Geometry check sheet. Reference: the model listing, model coordinates, mm. Face numbers are marked on the shaded views. A direction names the side the tool comes from. Give positions to 0.01 mm unless a question says otherwise; leave off trailing zeros. Loops run counter-clockwise (first coordinate to the right, second up) from the corner with the lowest first, then second, coordinate; pieces in that order, holes last. Notation, with made-up numbers: (-8, 21.25) - (18, 21.25) arc R19 cw to (18, 51.25) - close; hole circle Ø9 at (38, 4.5). An arc over 180 degrees is marked (long way). Use a Markdown table: item, result. Add a question column.
1. Depth check by flat-ended pin: P1, Ø17.5, axis at x = -1.5, y = 158.5, coming from the -Z side. Enter the tip coordinate at first touch or a pass-through.
2. Cross-section at B-B on x = -0.5. Enter the section's corners in (y, z), and give its area (3 significant figures).
3. Material ranges on L1, parallel to X at y = 82, z = -1.75; L2, parallel to Z at x = 1, y = 62; L3, parallel to X at y = 168.5, z = -6.5, recorded low to high.
4. Set-up check for the marked faces 1 and 2: record each of +Z, -Z, +X, -X, +Y, -Y from which the full face is reachable in a straight line by a thin tool's end or side.
5. Cross-section at A-A on y = 31.5. Enter the section's corners in (x, z).
from build123d import *

# Parameters (mm, degrees)
RUNDUNG_DEPTH        = 250
SKIZZE2_W            = 22
SKIZZE2_H            = 3.270726357
AUSSPARUNGLAUF_DEPTH = 252.122480077


with BuildPart() as part:
    # Skizze1 → Rundung (new body)
    with BuildSketch(Plane(origin=(0, 0, 0), x_dir=(1, 0, 0), z_dir=(0, 1, 0))):
        with BuildLine():
            Line((-19.158288024, 7.5), (-22.5, 7.5))
            Line((-22.5, 7.5), (-22.5, -7.5))
            Line((-22.5, -7.5), (22.5, -7.5))
            Line((22.5, -7.5), (22.5, 7.5))
            Line((22.5, 7.5), (19.158288024, 7.5))
            ThreePointArc((19.158288024, 7.5), (0, 1.3), (-19.158288024, 7.5))
        make_face()
    extrude(amount=RUNDUNG_DEPTH)

    # Skizze2 → AussparungLauf (cut, through all)
    with BuildSketch(Plane(origin=(0, 250, 0), x_dir=(1, 0, 0), z_dir=(0, 1, 0))):
        with Locations((0, 2.935363178)):
            Rectangle(SKIZZE2_W, SKIZZE2_H)
    extrude(amount=-AUSSPARUNGLAUF_DEPTH, mode=Mode.SUBTRACT)


solid = part.part
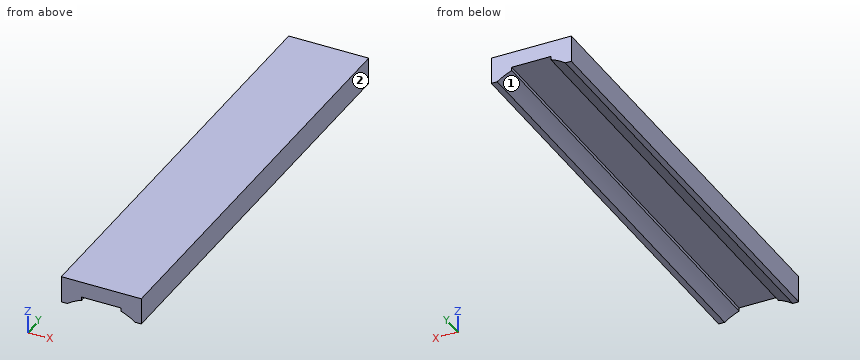
Values found:
| question | item | result |
|---|---|---|
| 1 | P1 | stops at z = -1.3 |
| 2 | outline | (0, -1.3) - (250, -1.3) - (250, 7.5) - (0, 7.5) - close |
| 2 | area | 2,200 mm2 |
| 3 | L1 | x = -22.5 to -11, 11 to 22.5 |
| 3 | L2 | z = -1.3 to 7.5 |
| 3 | L3 | x = -22.5 to -17.69, 17.69 to 22.5 |
| 4 | face 1 | -Z, +Y, -Y |
| 4 | face 2 | +Z, -Z, +X, +Y, -Y |
| 5 | outline | (-22.5, -7.5) - (-19.16, -7.5) arc R32.7 cw to (-11, -3.21) - (-11, -1.3) - (11, -1.3) - (11, -3.21) arc R32.7 cw to (19.16, -7.5) - (22.5, -7.5) - (22.5, 7.5) - (-22.5, 7.5) - close |
